from build123d import *

# Parameters (mm, degrees)
MAIN_DEPTH                     = 5.13
F_3_0_3_DIAMETER_HOLE2_D       = 3
F_3_0_3_DIAMETER_HOLE2_DEPTH   = 5.13
SKETCH4_W                      = 5.13
SKETCH4_H                      = 16.6
TEETH_HOLES_DEPTH              = 5.13
TEETH_HOLES_2_REACH            = 7.13
SKETCH5_W                      = 16.6
SKETCH5_H                      = 5.13
F_1_2_0_5_DIAMETER_HOLE1_D     = 12.7
F_1_2_0_5_DIAMETER_HOLE1_DEPTH = 5.13
M3_CLEARANCE_HOLE2_D           = 3.2
M3_CLEARANCE_HOLE2_DEPTH       = 5.08
M3_CLEARANCE_HOLE2_TIP         = 0.96137699


with BuildPart() as part:
    # Sketch1 → Main (new body)
    with BuildSketch(Plane(origin=(0, 0, 0), x_dir=(1, 0, 0), z_dir=(0, 1, 0))):
        with BuildLine():
            Line((-81.610197541, 55.143891453), (14.749802459, 55.143891453))
            ThreePointArc((14.749802459, 55.143891453), (15.456909241, 54.850998234), (15.749802459, 54.143891453))
            Line((15.749802459, 54.143891453), (15.749802459, -33.877426122))
            ThreePointArc((15.749802459, -33.877426122), (12.03005858, -42.857682243), (3.049802459, -46.577426122))
            Line((3.049802459, -46.577426122), (-69.910197541, -46.577426122))
            ThreePointArc((-69.910197541, -46.577426122), (-78.890453662, -42.857682243), (-82.610197541, -33.877426122))
            Line((-82.610197541, -33.877426122), (-82.610197541, 54.143891453))
            ThreePointArc((-82.610197541, 54.143891453), (-82.317304322, 54.850998234), (-81.610197541, 55.143891453))
        make_face()
    extrude(amount=MAIN_DEPTH)

    # Ø3.0 (3) Diameter Hole2
    with Locations(Plane(origin=(0, 5.13, 0), x_dir=(-1, 0, 0), z_dir=(0, 1, 0))):
        with Locations((55.020197541, -36.023891453), (11.840197541, -36.023891453), (55.020197541, 7.156108547), (11.840197541, 7.156108547)):
            Hole(F_3_0_3_DIAMETER_HOLE2_D / 2, depth=F_3_0_3_DIAMETER_HOLE2_DEPTH)

    # Sketch4 → Teeth holes (cut)
    with BuildSketch(Plane(origin=(0, 5.13, 0), x_dir=(1, 0, 0), z_dir=(0, 1, 0))):
        with Locations((-73.045197541, 25.708891453)):
            Rectangle(SKETCH4_W, SKETCH4_H)
        with Locations((6.184802459, 25.708891453)):
            Rectangle(SKETCH4_W, SKETCH4_H)
        with Locations((-73.045197541, -7.491108547)):
            Rectangle(SKETCH4_W, SKETCH4_H)
        with Locations((6.184802459, -7.491108547)):
            Rectangle(SKETCH4_W, SKETCH4_H)
    extrude(amount=-TEETH_HOLES_DEPTH, mode=Mode.SUBTRACT)

    # Sketch5 → Teeth holes 2 (cut, up to next)
    with BuildSketch(Plane(origin=(0, 5.13, 0), x_dir=(1, 0, 0), z_dir=(0, 1, 0)), mode=Mode.PRIVATE) as teeth_holes_2_sk1:
        with Locations((-50.030197541, 45.578891453)):
            Rectangle(SKETCH5_W, SKETCH5_H)
    teeth_holes_2_tool1 = extrude(teeth_holes_2_sk1.sketch, amount=-TEETH_HOLES_2_REACH, mode=Mode.PRIVATE) & part.part
    add(teeth_holes_2_tool1.solids().sort_by_distance((-50.030198, 5.13, -45.578891))[0], mode=Mode.SUBTRACT)
    # Sketch5 → Teeth holes 2 (cut, up to next)
    with BuildSketch(Plane(origin=(0, 5.13, 0), x_dir=(1, 0, 0), z_dir=(0, 1, 0)), mode=Mode.PRIVATE) as teeth_holes_2_sk2:
        with Locations((-16.830197541, 45.578891453)):
            Rectangle(SKETCH5_W, SKETCH5_H)
    teeth_holes_2_tool2 = extrude(teeth_holes_2_sk2.sketch, amount=-TEETH_HOLES_2_REACH, mode=Mode.PRIVATE) & part.part
    add(teeth_holes_2_tool2.solids().sort_by_distance((-16.830198, 5.13, -45.578891))[0], mode=Mode.SUBTRACT)
    # Sketch5 → Teeth holes 2 (cut, up to next)
    with BuildSketch(Plane(origin=(0, 5.13, 0), x_dir=(1, 0, 0), z_dir=(0, 1, 0)), mode=Mode.PRIVATE) as teeth_holes_2_sk3:
        with Locations((-50.030197541, -27.361108547)):
            Rectangle(SKETCH5_W, SKETCH5_H)
    teeth_holes_2_tool3 = extrude(teeth_holes_2_sk3.sketch, amount=-TEETH_HOLES_2_REACH, mode=Mode.PRIVATE) & part.part
    add(teeth_holes_2_tool3.solids().sort_by_distance((-50.030198, 5.13, 27.361109))[0], mode=Mode.SUBTRACT)
    # Sketch5 → Teeth holes 2 (cut, up to next)
    with BuildSketch(Plane(origin=(0, 5.13, 0), x_dir=(1, 0, 0), z_dir=(0, 1, 0)), mode=Mode.PRIVATE) as teeth_holes_2_sk4:
        with Locations((-16.830197541, -27.361108547)):
            Rectangle(SKETCH5_W, SKETCH5_H)
    teeth_holes_2_tool4 = extrude(teeth_holes_2_sk4.sketch, amount=-TEETH_HOLES_2_REACH, mode=Mode.PRIVATE) & part.part
    add(teeth_holes_2_tool4.solids().sort_by_distance((-16.830198, 5.13, 27.361109))[0], mode=Mode.SUBTRACT)

    # 1/2 (0.5) Diameter Hole1
    with Locations(Plane(origin=(0, 5.13, 0), x_dir=(-1, 0, 0), z_dir=(0, 1, 0))):
        with Locations((33.430197541, -14.433891453)):
            Hole(F_1_2_0_5_DIAMETER_HOLE1_D / 2, depth=F_1_2_0_5_DIAMETER_HOLE1_DEPTH)

    # M3 Clearance Hole2
    with Locations(Plane(origin=(0, 5.13, 0), x_dir=(-1, 0, 0), z_dir=(0, 1, 0))):
        with Locations((73.045197541, -9.108891453), (-6.184802459, -9.108891453), (33.430197541, 27.361108547)):
            Hole(M3_CLEARANCE_HOLE2_D / 2, depth=M3_CLEARANCE_HOLE2_DEPTH)
            with Locations((0, 0, -(M3_CLEARANCE_HOLE2_DEPTH + M3_CLEARANCE_HOLE2_TIP / 2))):  # 118° drill point
                Cone(0, M3_CLEARANCE_HOLE2_D / 2, M3_CLEARANCE_HOLE2_TIP, mode=Mode.SUBTRACT)


solid = part.part
Model file for the job. Use its own axes, mm. A direction names the side the tool comes from. Give positions to 0.01 mm unless a question says otherwise; leave off trailing zeros. Write each loop counter-clockwise with the first axis right and the second up, starting at its lowest first coordinate (ties: lowest second). Pieces come first, ordered by that corner, then holes. Notation, with made-up numbers: (-36, 3) -> (6, 3) arc R22 cw to (6, 9) -> close; hole circle Ø4 at (-15, 52.5). An arc over 180 degrees is marked (long way). Write item = value, one per line.
(1) Slice it at A-A, the plane z = 2. Give the cut face in (x, y).
Determined:
outline = (-82.61, 0) -> (-75.61, 0) -> (-75.61, 5.13) -> (-82.61, 5.13) -> close; (-70.48, 0) -> (3.62, 0) -> (3.62, 5.13) -> (-70.48, 5.13) -> close; (8.75, 0) -> (15.75, 0) -> (15.75, 5.13) -> (8.75, 5.13) -> close
(2) Mould opens along X. For faces 3 (the face through (-33, 0, -5)), 4 (the face through (3.62, 3, -26)), 5 (the face through (12.128, 2.529, 42.758)) say: released by +X, released by -X, zero draft, split by the parting line, or undercut.
Determined:
face_3 = zero draft
face_4 = undercut
face_5 = released by +X
(3) Slice it at B-B, the plane x = -16. Give the cut face in (y, z), then the cut area to 3 significant figures.
Determined:
outline = (0, -55.14) -> (5.13, -55.14) -> (5.13, -48.14) -> (0, -48.14) -> close; (0, -43.01) -> (5.13, -43.01) -> (5.13, 24.8) -> (0, 24.8) -> close; (0, 29.93) -> (5.13, 29.93) -> (5.13, 46.58) -> (0, 46.58) -> close
area = 469 mm2
(4) Slice it at C-C, the plane x = -55. Give the cut face in (y, z), then the cut area to 3 significant figures.
Determined:
outline = (0, -55.14) -> (5.13, -55.14) -> (5.13, -48.14) -> (0, -48.14) -> close; (0, -43.01) -> (5.13, -43.01) -> (5.13, -37.52) -> (0, -37.52) -> close; (0, -34.52) -> (5.13, -34.52) -> (5.13, 5.66) -> (0, 5.66) -> close; (0, 8.66) -> (5.13, 8.66) -> (5.13, 24.8) -> (0, 24.8) -> close; (0, 29.93) -> (5.13, 29.93) -> (5.13, 46.58) -> (0, 46.58) -> close
area = 438 mm2
(5) Probe line 1 along X through (y, z) = (1.7, -24); line 2 along Z through (x, y) = (-49, 2.4); line 3 along X through (y, z) = (1.95, 25). List the from-to ranges inside material, lowest first.
Determined:
line_1 = -82.61 to -75.61, -70.48 to 3.62, 8.75 to 15.75
line_2 = -55.14 to -48.14, -43.01 to 24.8, 29.93 to 46.58
line_3 = -82.61 to -58.33, -41.73 to -25.13, -8.53 to 15.75
(6) Slice it at D-D, the plane z = -19. Give the cut face in (x, y), then the cut area to 3 significant figures.
Determined:
outline = (-82.61, 0) -> (-75.61, 0) -> (-75.61, 5.13) -> (-82.61, 5.13) -> close; (-70.48, 0) -> (-37.84, 0) -> (-37.84, 5.13) -> (-70.48, 5.13) -> close; (-29.02, 0) -> (3.62, 0) -> (3.62, 5.13) -> (-29.02, 5.13) -> close; (8.75, 0) -> (15.75, 0) -> (15.75, 5.13) -> (8.75, 5.13) -> close
area = 407 mm2
(7) Tool access for faces 1 (the face through (15.75, 3, -11)), 2 (the face through (-41.73, 3, 27)): list every direction of +Z, -Z, +X, -X, +Y, -Y with a clear straight run to the whole face (end or side of a thin tool).
Determined:
face_1 = +Z, -Z, +X, +Y, -Y
face_2 = +Y, -Y
